The drawing under review shows one solid part. Ordinate dimensions are in mm from its lowest x, y, z. Coordinates: 2 decimals unless noted, no trailing zeros. Write each loop counter-clockwise with the first axis right and the second up, starting at its lowest first coordinate (ties: lowest second). Pieces come first, ordered by that corner, then holes. Notation, with made-up numbers: (6, 80) -> (43, 80) arc R19 cw to (43, 85) -> close; hole circle Ø3 at (37.5, -18.75). An arc over 180 degrees is marked (long way). Put each result on its own line as item: value. Start each with the question number.
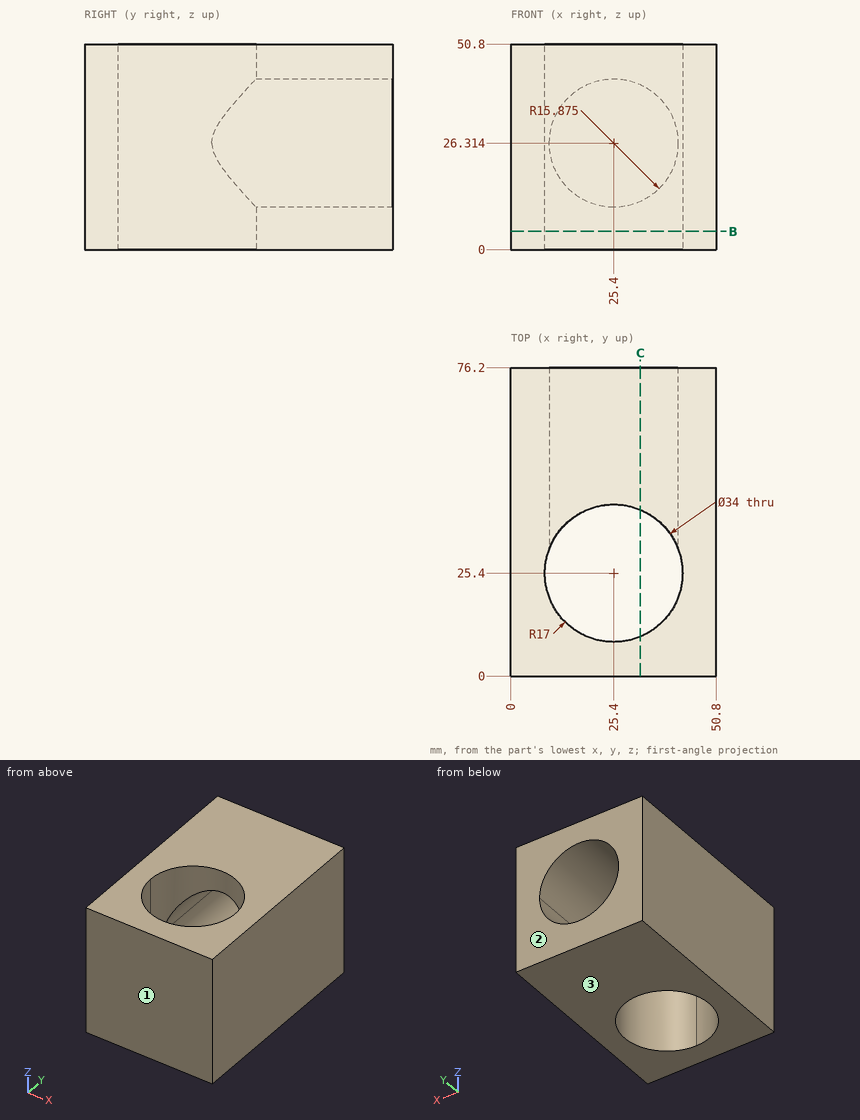
1. Consider section C-C on x = 32. State the section outline as (y, z) points, then the cut area to 3 significant figures.
2. Wall thickness on line 1 (X direction, y = 25.4, z = 11); line 2 (X direction, y = 41.5, z = 26); line 3 (Z direction, x = 39, y = 71) (1 decimal): over which ranges is each line inside the solid? List them lowest first. Write a range as from..to.
3. The part is to be moulded in two halves that separate along Y. For the marked faces 1, 2 and 3, say which applies: released by +Y, released by -Y, zero draft, split by the parting line, or undercut.
4. Insertion check: P1, Ø6, axis at x = 19, z = 25.5, coming from the +Y side (1 decimal); P2, Ø8, axis at x = 28, z = 31.5, coming from the +Y side; P3, Ø5, axis at x = 28, z = 29, coming from the +Y side. Each pin has a flat end and moves straight along its axis. Give the tip position at first contact, or say it passes through.
5. Consider section B-B on z = 4.5. State the section outline as (x, y) points.
Output values:
1. outline: (0, 0) -> (9.73, 0) -> (9.73, 50.8) -> (0, 50.8) -> close; (41.07, 0) -> (76.2, 0) -> (76.2, 11.88) -> (41.07, 11.88) -> close; (41.07, 40.75) -> (76.2, 40.75) -> (76.2, 50.8) -> (41.07, 50.8) -> close
1. area: 1,260 mm^2
2. line 1: x = 0..8.4, 42.4..50.8
2. line 2: x = 0..9.53, 41.27..50.8
2. line 3: z = 0..18.1, 34.5..50.8
3. face 1: released by -Y
3. face 2: released by +Y
3. face 3: zero draft
4. P1: stops at y = 11.2
4. P2: stops at y = 9.73
4. P3: stops at y = 9.18
5. outline: (0, 0) -> (50.8, 0) -> (50.8, 76.2) -> (0, 76.2) -> close; hole circle Ø34 at (25.4, 25.4)
